Geometry check sheet. Reference: the model listing, model coordinates, mm. Face numbers are marked on the shaded views. A direction names the side the tool comes from. Coordinates: 2 decimals unless noted, no trailing zeros. Order: outer loops, then holes, each group sorted by start corner. A loop starts at its lowest first (then second) coordinate and runs counter-clockwise, first axis right, second up. Notation, with made-up numbers: (50.25, -29) -> (98.25, -29) arc R34 ccw to (98.25, 9) -> close; hole circle Ø1 at (38, 89.25). An arc over 180 degrees is marked (long way). Answer in a Markdown table with one row per item. Add a question column.
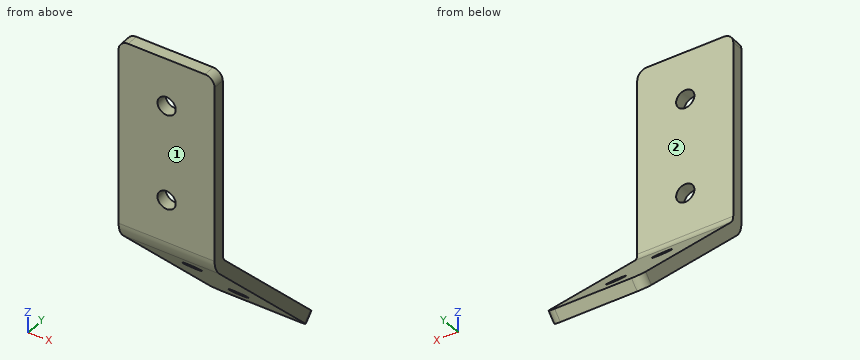
```python
from build123d import *

# Parameters (mm, degrees)
BOSS_EXTRUDE1_DEPTH    = 25.4
CUT_EXTRUDE1_REACH     = 101.249
SKETCH2_R              = 2.413
CUT_EXTRUDE2_REACH     = 96.062
SKETCH3_R              = 2.413
CONVERT_SOLID1_DEPTH   = 25.4
CONVERT_SOLID1_2_DEPTH = 25.4
FILLET1_R              = 2.54


# Read off the part's stored shape, not the designer's step: Convert-Solid1
with BuildPart() as part:
    # Sketch1 → Boss-Extrude1 (new body)
    with BuildSketch(Plane(origin=(0, 0, 0), x_dir=(0, 0, -1), z_dir=(1, 0, 0))):
        Polygon((0, 0), (52.115128061, 0), (88.966088515, 36.850960454), (86.721024484, 39.096024484), (50.8, 3.175), (0, 3.175), align=None)
    extrude(amount=BOSS_EXTRUDE1_DEPTH)

    # Sketch2 → Cut-Extrude1 (cut, up to next)
    with BuildSketch(Plane(origin=(0, 3.175, 0), x_dir=(1, 0, 0), z_dir=(0, 1, 0)), mode=Mode.PRIVATE) as cut_extrude1_sk1:
        with Locations(Location((12.7, 12.7, 0), (0, 0, 270))):
            Circle(SKETCH2_R)
    cut_extrude1_tool1 = extrude(cut_extrude1_sk1.sketch, amount=-CUT_EXTRUDE1_REACH, mode=Mode.PRIVATE) & part.part
    # Sketch2 → Cut-Extrude1 (cut, up to next)
    with BuildSketch(Plane(origin=(0, 3.175, 0), x_dir=(1, 0, 0), z_dir=(0, 1, 0)), mode=Mode.PRIVATE) as cut_extrude1_sk2:
        with Locations(Location((12.7, 38.1, 0), (0, 0, 270))):
            Circle(SKETCH2_R)
    cut_extrude1_tool2 = extrude(cut_extrude1_sk2.sketch, amount=-CUT_EXTRUDE1_REACH, mode=Mode.PRIVATE) & part.part
    add(cut_extrude1_tool1.solids().sort_by_distance((12.7, 3.175, -12.7))[0], mode=Mode.SUBTRACT)
    add(cut_extrude1_tool2.solids().sort_by_distance((12.7, 3.175, -38.1))[0], mode=Mode.SUBTRACT)

    # Sketch3 → Cut-Extrude2 (cut, up to next)
    with BuildSketch(Plane(origin=(0, -23.8125, -23.8125), x_dir=(1, 0, 0), z_dir=(0, 0.707106781186546, 0.707106781186549)), mode=Mode.PRIVATE) as cut_extrude2_sk1:
        with Locations(Location((12.7, 76.266088515, 0), (0, 0, 270))):
            Circle(SKETCH3_R)
    cut_extrude2_tool1 = extrude(cut_extrude2_sk1.sketch, amount=-CUT_EXTRUDE2_REACH, mode=Mode.PRIVATE) & part.part
    # Sketch3 → Cut-Extrude2 (cut, up to next)
    with BuildSketch(Plane(origin=(0, -23.8125, -23.8125), x_dir=(1, 0, 0), z_dir=(0, 0.707106781186546, 0.707106781186549)), mode=Mode.PRIVATE) as cut_extrude2_sk2:
        with Locations(Location((12.7, 50.866088515, 0), (0, 0, 270))):
            Circle(SKETCH3_R)
    cut_extrude2_tool2 = extrude(cut_extrude2_sk2.sketch, amount=-CUT_EXTRUDE2_REACH, mode=Mode.PRIVATE) & part.part
    add(cut_extrude2_tool1.solids().sort_by_distance((12.7, 30.115768, -77.740768))[0], mode=Mode.SUBTRACT)
    add(cut_extrude2_tool2.solids().sort_by_distance((12.7, 12.155256, -59.780256))[0], mode=Mode.SUBTRACT)

    # Convert-Solid1 outline → Convert-Solid1 (cut)
    with BuildSketch(Plane.YZ):
        with BuildLine():
            Line((0, -52.115128061), (1.859871939, -53.975))
            ThreePointArc((1.859871939, -53.975), (0.483364969, -51.914911734), (0, -49.484871939))
            Line((0, -49.484871939), (0, -52.115128061))
        make_face()
    extrude(amount=CONVERT_SOLID1_DEPTH, mode=Mode.SUBTRACT)

    # Convert-Solid1 2 outline → Convert-Solid1 2 (add)
    with BuildSketch(Plane.YZ):
        with BuildLine():
            Line((3.175, -50.8), (4.10493597, -51.72993597))
            ThreePointArc((4.10493597, -51.72993597), (3.416682484, -50.699891837), (3.175, -49.484871939))
            Line((3.175, -49.484871939), (3.175, -50.8))
        make_face()
    extrude(amount=CONVERT_SOLID1_2_DEPTH)

    # Fillet1
    fillet1_edges = [part.edges().sort_by_distance(p)[0] for p in [
        (0, 1.5875, 0),
        (25.4, 1.5875, 0),
        (25.4, 37.973492469, -87.843556499),
        (0, 37.973492469, -87.843556499),
    ]]
    fillet(fillet1_edges, radius=FILLET1_R)


solid = part.part
```
(1) Cross-section at C-C (x = 12.7). Give the number of separate pieces and of enclosed holes in the cut face, plus the area to 3 significant figures.
(2) Cross-section at B-B (x = 8.5). Enter the section's corners in (y, z) (3 decimals).
(3) Scan lines: line 1 along X through (y, z) = (0.95, -38.1); line 2 along Y through (x, z) = (20, -39.5) (3 decimals); line 3 along X through (y, z) = (1, -12). Record each from-to range of solid material in increasing order.
(4) Cross-section at A-A (z = -38.1). Enter the section's corners in (x, y) (3 decimals).
(5) Go/stop test with flat-tipped pins: P1, Ø4, axis at x = 15.5, z = -29.5, coming from the +Y side (3 decimals); P2, Ø8, axis at x = 12, y = 26, coming from the +Z side (3 decimals); P3, Ø4, axis at x = 12.7, z = -12.7, coming from the -Y side; P4, Ø12, axis at x = 13, y = 28.5, coming from the +Z side (3 decimals). Record where each tip stops, or that it passes through.
(6) Cross-section at D-D (z = -66). Enter the section's corners in (x, y) (3 decimals).
(7) Access from +Z, -Z, +X, -X, +Y, -Y to the whole of each face (thin tool, end or side, straight path). Record for the marked faces 1 and 2.
Checks:
| question | item | result |
|---|---|---|
| 1 | separate pieces | 5 |
| 1 | enclosed holes | 0 |
| 1 | area | 265 mm² |
| 2 | outline | (0, -49.485) arc R6.35 ccw to (1.86, -53.975) -> (36.851, -88.966) -> (39.096, -86.721) -> (4.105, -51.73) arc R3.175 cw to (3.175, -49.485) -> (3.175, 0) -> (0, 0) -> close |
| 3 | line 1 | 0 to 10.29, 15.11 to 25.4 |
| 3 | line 2 | 0 to 3.175 |
| 3 | line 3 | 0 to 10.39, 15.01 to 25.4 |
| 4 | outline | (0, 0) -> (10.287, 0) -> (10.287, 3.175) -> (0, 3.175) -> close; (15.113, 0) -> (25.4, 0) -> (25.4, 3.175) -> (15.113, 3.175) -> close |
| 5 | P1 | y = 3.175 |
| 5 | P2 | z = -69.625 |
| 5 | P3 | through |
| 5 | P4 | z = -70.125 |
| 6 | outline | (0, 13.885) -> (25.4, 13.885) -> (25.4, 18.375) -> (0, 18.375) -> close |
| 7 | face 1 | +Z, -Z, +X, -X, -Y |
| 7 | face 2 | +Z, +X, -X, +Y |
